Could you check a few things on this model? Use its own coordinates, in mm. Give positions to 0.01 mm unless a question says otherwise; leave off trailing zeros. Loops run counter-clockwise (first coordinate to the right, second up) from the corner with the lowest first, then second, coordinate; pieces in that order, holes last. Notation, with made-up numbers: (-20.75, 20.25) - (30.25, 20.25) arc R23 cw to (30.25, 53.25) - close; hole circle Ø1 at (32, 59.25). An arc over 180 degrees is marked (long way). Write each question's results on one line, items separated by ' | '. Start each with the question number.
(1) Suppose I cut it at A-A (y = 69). Please give me the cut outline in (x, z).
(2) For pin 1 (1 mm diameter, centred on x = -6.5, y = 54.5, fed in from +Z); pin 2 (1 mm diameter, centred on x = 3.5, z = 1, fed in from +Y); pin 3 (1.5 mm diameter, centred on x = 3, y = 89.5, fed in from -Z), each with a flat end and sliding along its axis, tell me the tip position at first contact or that it passes through.
(3) I need wall thicknesses on line 1 (Y direction, x = -3.5, z = 6.75); line 2 (Z direction, x = 0.5, y = 65); line 3 (X direction, y = 37.5, z = -10). Which ranges of each line are inside material? Lowest first, please.
from build123d import *

# Parameters (mm, degrees)
SKETCH2_R           = 15
BOSS_EXTRUDE1_DEPTH = 100
CHAMFER1_SIZE       = 25
CHAMFER1_SIZE2      = 6.698729811
SKETCH3_R           = 0.5
BOSS_EXTRUDE2_DEPTH = 5


with BuildPart() as part:
    # Sketch2 → Boss-Extrude1 (new body)
    with BuildSketch(Plane(origin=(0, 0, 0), x_dir=(1, 0, 0), z_dir=(0, 1, 0))):
        Circle(SKETCH2_R)
    extrude(amount=BOSS_EXTRUDE1_DEPTH)

    # Chamfer1
    chamfer1_edges = [part.edges().sort_by_distance(p)[0] for p in [
        (-15, 0, 0),
    ]]
    chamfer1_side = [part.faces().sort_by_distance(p)[0] for p in [
        (-15, 50, 0),
    ]]
    chamfer(chamfer1_edges, length=CHAMFER1_SIZE, length2=CHAMFER1_SIZE2, reference=chamfer1_side[0])

    # Sketch3 → Boss-Extrude2 (add)
    with BuildSketch(Plane(origin=(0, 100, 0), x_dir=(1, 0, 0), z_dir=(0, 1, 0))):
        Circle(SKETCH3_R)
    extrude(amount=BOSS_EXTRUDE2_DEPTH)


solid = part.part
Output values:
1) outline: circle Ø30 at (0, 0)
2) pin 1: z = 13.75 | pin 2: y = 100 | pin 3: z = -14.83
3) line 1: 0 to 100 | line 2: -14.99 to 14.99 | line 3: -11.18 to 11.18
